from build123d import *

# Parameters (mm, degrees)
CYLINDER_R        = 20
CYLINDER_DEPTH    = 34
CYLINDER001_R     = 5.5
CYLINDER001_DEPTH = 32
FILLET_R          = 1
FILLET001_R       = 0.4


with BuildPart() as part:
    # Cylinder → Cylinder (join)
    with BuildSketch(Plane.XY):
        Circle(CYLINDER_R)
    extrude(amount=CYLINDER_DEPTH)

    # Cylinder001 → Cylinder001 (cut)
    with BuildSketch(Plane(origin=(0, 0, 34), x_dir=(-1, 0, 0), z_dir=(0, 0, -1))):
        Circle(CYLINDER001_R)
    extrude(amount=CYLINDER001_DEPTH, mode=Mode.SUBTRACT)

    # Cone → Cone (revolve, cut)
    with BuildSketch(Plane(origin=(0, 0, 34), x_dir=(-1, 0, 0), z_dir=(0, -1, 0))):
        Polygon((0, 0), (9.5, 0), (7.5, 5), (0, 5), align=None)
    revolve(axis=Axis((0, 0, 34), (0, 0, -1)), mode=Mode.SUBTRACT)

    # Fillet
    fillet_edges = [part.edges().sort_by_distance(p)[0] for p in [
        (-20, 0, 34),
        (9.5, 0, 34),
        (5.5, 0, 29),
        (5.5, 0, 2),
    ]]
    fillet(fillet_edges, radius=FILLET_R)

    # Fillet001
    fillet001_edges = [part.edges().sort_by_distance(p)[0] for p in [
        (-20, 0, 0),
    ]]
    fillet(fillet001_edges, radius=FILLET001_R)


solid = part.part
Check sheet for the modelled part. Datum: model origin and axes. Units: mm. A direction names the side the tool comes from. Round coordinates to 2 decimals unless told otherwise and drop trailing zeros. Loops run counter-clockwise (first coordinate to the right, second up) from the corner with the lowest first, then second, coordinate; pieces in that order, holes last. Notation, with made-up numbers: M -24,61.5 L 25,61.5 A23 cw 25,97.5 Z; hole C -25.5,37.5 d6. An arc over 180 degrees is marked long. One line per item, written item: value.
(1) Sectioned sample at D-D, the plane z = 31. Record the cut outline in (x, y).
Computed values:
outline: C 0,0 d40; hole C 0,0 d16.6
(2) Depth check by flat-ended pin: pin 1 Ø5 at (x, y) = (6, 4.5) entering from +Z; pin 2 Ø2.5 at (x, y) = (1.5, -1) entering from +Z; pin 3 Ø12 at (x, y) = (1, -1) entering from +Z. Enter the tip coordinate at first touch or a pass-through.
Computed values:
pin 1: stops at z = 33.98
pin 2: stops at z = 2
pin 3: stops at z = 29
(3) Sectioned sample at A-A, the plane x = 0. Record the cut outline in (y, z), then the cut area to 3 significant figures.
Computed values:
outline: M -20,0.4 A0.4 ccw -19.6,0 L 19.6,0 A0.4 ccw 20,0.4 L 20,33 A1 ccw 19,34 L 10.18,34 A1 ccw 9.25,33.37 L 7.5,29 L 6.5,29 A1 ccw 5.5,28 L 5.5,3 A1 cw 4.5,2 L -4.5,2 A1 cw -5.5,3 L -5.5,28 A1 ccw -6.5,29 L -7.5,29 L -9.25,33.37 A1 ccw -10.18,34 L -19,34 A1 ccw -20,33 Z
area: 977 mm^2
(4) Release check for a two-part mould opening along Y. For faces 1 (the face through (-4.336, -19.524, 16.472)), 2 (the face through (0, 0, 0)), 3 (the face through (0, 0, 2)) record: +Y half, -Y half, draft (parallel to the pull), parting line (faces both ways), or undercut.
Computed values:
face 1: parting line
face 2: draft
face 3: undercut
(5) Sectioned sample at C-C, the plane z = 21. Record the cut outline in (x, y).
Computed values:
outline: C 0,0 d40; hole C 0,0 d11
(6) Access from +Z, -Z, +X, -X, +Y, -Y to the whole of each face (thin tool, end or side, straight path). Record for faces 4 (the face through (1.19, -5.37, 15.68)), 5 (the face through (8, -8, 34)).
Computed values:
face 4: +Z
face 5: +Z, +X, -X, +Y, -Y
(7) Thickness scan on line 1 (Y direction, x = 0, z = 16.5); line 2 (Y direction, x = 2, z = 8); line 3 (X direction, y = 5, z = 4). Record the ranges inside material, lowest first.
Computed values:
line 1: y = -20 to -5.5, 5.5 to 20
line 2: y = -19.9 to -5.12, 5.12 to 19.9
line 3: x = -19.36 to -2.29, 2.29 to 19.36
